```python
from build123d import *

# Parameters (mm, degrees)
SKETCH1_R           = 15
SKETCH1_R_2         = 13
BOSS_EXTRUDE1_DEPTH = 2
BOSS_EXTRUDE2_START = 1
SKETCH2_R           = 15
BOSS_EXTRUDE2_DEPTH = 1
FILLET1_R           = 0.5


with BuildPart() as part:
    # Sketch1 → Boss-Extrude1 (new body)
    with BuildSketch(Plane.XY):
        Circle(SKETCH1_R)
        Circle(SKETCH1_R_2, mode=Mode.SUBTRACT)
    extrude(amount=BOSS_EXTRUDE1_DEPTH)

    # Sketch2 → Boss-Extrude2 (add)
    with BuildSketch(Plane(origin=(0, 0, 0), x_dir=(-1, 0, 0), z_dir=(0, 0, -1)).offset(BOSS_EXTRUDE2_START)):
        Circle(SKETCH2_R)
    extrude(amount=-BOSS_EXTRUDE2_DEPTH)

    # Fillet1
    fillet1_edges = [part.edges().sort_by_distance(p)[0] for p in [
        (15, 0, -1),
    ]]
    fillet(fillet1_edges, radius=FILLET1_R)


solid = part.part
```
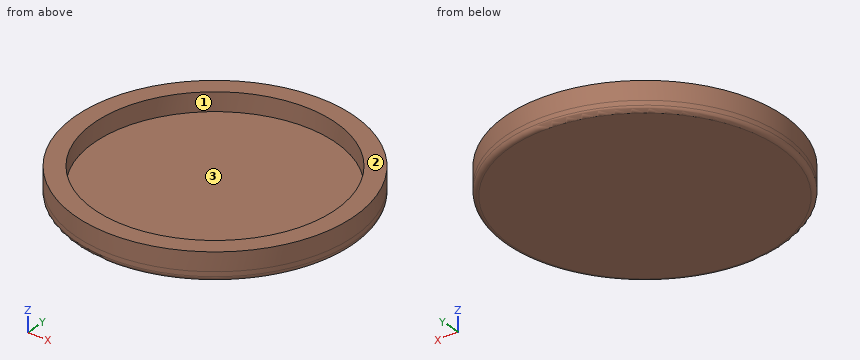
Design review of the part built by this model. Coordinates are the model's own, in mm. Face numbers are marked on the shaded views. Coordinates: 2 decimals unless noted, no trailing zeros. Order: outer loops, then holes, each group sorted by start corner. A loop starts at its lowest first (then second) coordinate and runs counter-clockwise, first axis right, second up. Notation, with made-up numbers: M 12.25,65.25 L 17.25,65.25 A31 ccw 17.25,93.25 Z; hole C 51.25,-38.5 d3. An arc over 180 degrees is marked long. Answer as a JSON object with one key per item and string values. Group by question number.
1) For pin 1 (10 mm diameter, centred on x = -2.5, y = -2, fed in from +Z), flat-tipped, find the tip position at first contact; note if it passes through.
2) Add section A-A, the plane y = 0. Write out the cut boundary in (x, z), then the cut area to 3 significant figures.
3) Mouldability with a two-part tool opening along Y and no side actions: class the marked faces 1, 2 and 3 as pulls with the +Y half, pulls with the -Y half, needs draft (parallel to the pull), parting line crosses it, or undercut.
4) Add section C-C, the plane z = 0.5. Write out the cut boundary in (x, y).
5) Wall thickness on L1, parallel to Y at x = 0, z = 1.2; L2, parallel to Z at x = 7.5, y = -5; L3, parallel to Y at x = -8.5, z = 0.65: over which ranges is each line inside the solid? List them lowest first.
Computed values:
{
 "1": {"pin 1": "stops at z = 0"},
 "2": {"outline": "M -15,-0.5 A0.5 ccw -14.5,-1 L 14.5,-1 A0.5 ccw 15,-0.5 L 15,2 L 13,2 L 13,0 L -13,0 L -13,2 L -15,2 Z", "area": "37.9 mm^2"},
 "3": {"face 1": "undercut", "face 2": "needs draft", "face 3": "undercut"},
 "4": {"outline": "C 0,0 d30; hole C 0,0 d26"},
 "5": {"L1": "y = -15 to -13, 13 to 15", "L2": "z = -1 to 0", "L3": "y = -12.36 to -9.84, 9.84 to 12.36"}
}
